The listing builds one solid part. Answer for the finished solid, in the listing's coordinates (mm). A direction names the side the tool comes from. Give positions to 0.01 mm unless a question says otherwise; leave off trailing zeros. Order: outer loops, then holes, each group sorted by start corner. A loop starts at its lowest first (then second) coordinate and runs counter-clockwise, first axis right, second up.
```python
from build123d import *

# Parameters (mm, degrees)
SKETCH2_W                  = 125
SKETCH2_H                  = 95
SKETCH2_R                  = 8
BOSS_EXTRUDE1_DEPTH        = 30
SKETCH3_W                  = 60
SKETCH3_H                  = 60
CUT_EXTRUDE1_DEPTH         = 20
SKETCH4_R                  = 25.5
CUT_EXTRUDE2_DEPTH         = 82.00925873
FILLET1_R                  = 7
FILLET3_R                  = 3
M4_CLEARANCE_HOLE1_D       = 4.5
M6X1_0_TAPPED_HOLE1_REACH  = 119.606
M6X1_0_TAPPED_HOLE1_BORE_R = 2.5
M6X1_0_TAPPED_HOLE2_REACH  = 119.606
M6X1_0_TAPPED_HOLE2_BORE_R = 2.5


with BuildPart() as part:
    # Sketch2 → Boss-Extrude1 (new body)
    with BuildSketch(Plane(origin=(0, 0, 0), x_dir=(1, 0, 0), z_dir=(0, 1, 0))):
        Rectangle(SKETCH2_W, SKETCH2_H)
        with Locations(Location((-44, 29, 0), (0, 0, 270))):
            Circle(SKETCH2_R, mode=Mode.SUBTRACT)
        with Locations(Location((-44, -29, 0), (0, 0, 270))):
            Circle(SKETCH2_R, mode=Mode.SUBTRACT)
        with Locations(Location((44, -29, 0), (0, 0, 270))):
            Circle(SKETCH2_R, mode=Mode.SUBTRACT)
        with Locations(Location((44, 29, 0), (0, 0, 270))):
            Circle(SKETCH2_R, mode=Mode.SUBTRACT)
    extrude(amount=BOSS_EXTRUDE1_DEPTH)

    # Sketch3 → Cut-Extrude1 (cut)
    with BuildSketch(Plane(origin=(0, 30, 0), x_dir=(1, 0, 0), z_dir=(0, 1, 0))):
        Rectangle(SKETCH3_W, SKETCH3_H)
    extrude(amount=-CUT_EXTRUDE1_DEPTH, mode=Mode.SUBTRACT)

    # Sketch4 → Cut-Extrude2 (cut, through all)
    with BuildSketch(Plane(origin=(0, 10, 0), x_dir=(1, 0, 0), z_dir=(0, 1, 0))):
        with Locations(Location((0, 0, 0), (0, 0, 270))):
            Circle(SKETCH4_R)
    extrude(amount=-CUT_EXTRUDE2_DEPTH, mode=Mode.SUBTRACT)

    # Fillet1
    fillet1_edges = [part.edges().sort_by_distance(p)[0] for p in [
        (30, 20, -30),
        (30, 20, 30),
        (-30, 20, 30),
        (-30, 20, -30),
    ]]
    fillet(fillet1_edges, radius=FILLET1_R)

    # Fillet3
    fillet3_edges = [part.edges().sort_by_distance(p)[0] for p in [
        (-62.5, 15, -47.5),
        (62.5, 15, -47.5),
        (62.5, 15, 47.5),
        (-62.5, 15, 47.5),
    ]]
    fillet(fillet3_edges, radius=FILLET3_R)

    # M4 Clearance Hole1 (through all)
    with Locations(Plane(origin=(0, 30, 0), x_dir=(1, 0, 0), z_dir=(0, 1, 0))):
        with Locations((-22, 22), (22, 22), (22, -22), (-22, -22)):
            Hole(M4_CLEARANCE_HOLE1_D / 2)

    # M6x1.0 Tapped Hole1 bore → M6x1.0 Tapped Hole1 (cut, up to next)
    with BuildSketch(Plane.XY.offset(47.5), mode=Mode.PRIVATE) as m6x1_0_tapped_hole1_sk1:
        with Locations((-44, 15)):
            Circle(M6X1_0_TAPPED_HOLE1_BORE_R)
    m6x1_0_tapped_hole1_tool1 = extrude(m6x1_0_tapped_hole1_sk1.sketch, amount=-M6X1_0_TAPPED_HOLE1_REACH, mode=Mode.PRIVATE) & part.part
    # M6x1.0 Tapped Hole1 bore → M6x1.0 Tapped Hole1 (cut, up to next)
    with BuildSketch(Plane.XY.offset(47.5), mode=Mode.PRIVATE) as m6x1_0_tapped_hole1_sk2:
        with Locations((44, 15)):
            Circle(M6X1_0_TAPPED_HOLE1_BORE_R)
    m6x1_0_tapped_hole1_tool2 = extrude(m6x1_0_tapped_hole1_sk2.sketch, amount=-M6X1_0_TAPPED_HOLE1_REACH, mode=Mode.PRIVATE) & part.part
    add(m6x1_0_tapped_hole1_tool1.solids().sort_by_distance((-44, 15, 47.5))[0], mode=Mode.SUBTRACT)
    add(m6x1_0_tapped_hole1_tool2.solids().sort_by_distance((44, 15, 47.5))[0], mode=Mode.SUBTRACT)

    # M6x1.0 Tapped Hole2 bore → M6x1.0 Tapped Hole2 (cut, up to next)
    with BuildSketch(Plane(origin=(0, 0, -47.5), x_dir=(-1, 0, 0), z_dir=(0, 0, -1)), mode=Mode.PRIVATE) as m6x1_0_tapped_hole2_sk1:
        with Locations((-44, 15)):
            Circle(M6X1_0_TAPPED_HOLE2_BORE_R)
    m6x1_0_tapped_hole2_tool1 = extrude(m6x1_0_tapped_hole2_sk1.sketch, amount=-M6X1_0_TAPPED_HOLE2_REACH, mode=Mode.PRIVATE) & part.part
    # M6x1.0 Tapped Hole2 bore → M6x1.0 Tapped Hole2 (cut, up to next)
    with BuildSketch(Plane(origin=(0, 0, -47.5), x_dir=(-1, 0, 0), z_dir=(0, 0, -1)), mode=Mode.PRIVATE) as m6x1_0_tapped_hole2_sk2:
        with Locations((44, 15)):
            Circle(M6X1_0_TAPPED_HOLE2_BORE_R)
    m6x1_0_tapped_hole2_tool2 = extrude(m6x1_0_tapped_hole2_sk2.sketch, amount=-M6X1_0_TAPPED_HOLE2_REACH, mode=Mode.PRIVATE) & part.part
    add(m6x1_0_tapped_hole2_tool1.solids().sort_by_distance((44, 15, -47.5))[0], mode=Mode.SUBTRACT)
    add(m6x1_0_tapped_hole2_tool2.solids().sort_by_distance((-44, 15, -47.5))[0], mode=Mode.SUBTRACT)


solid = part.part
```
1) Straight lines are drawn through the part: probe 1 along X at (y, z) = (15, 42); probe 2 along Z at (x, y) = (-22, 3.5); probe 3 along X at (y, z) = (2, -30). For each, find the intervals that lie inside material, in ascending order.
Geometry says:
probe 1: x = -62.5 to -46.5, -41.5 to 41.5, 46.5 to 62.5
probe 2: z = -47.5 to -24.25, -19.75 to -12.89, 12.89 to 19.75, 24.25 to 47.5
probe 3: x = -62.5 to -51.94, -36.06 to 36.06, 51.94 to 62.5
2) A tool of negligible diameter and unlimited length cuts with its end or side. For faces 4 (the flat face through (30, 20, 0)), 5 (the cylindrical face through (20.962, 4.93, 23.996)), 6 (the cylindrical face through (41.69, 14.04, -42.13)), 7 (the flat face through (-1, 15, 47.5)), 8 (the cylindrical face through (46.31, 14.04, 42.13)), from which of +Z, -Z, +X, -X, +Y, -Y can it reach the whole face along a straight path? Write none if from no direction.
Geometry says:
face 4: +Y
face 5: +Y, -Y
face 6: -Z
face 7: +Z, +X, -X, +Y, -Y
face 8: +Z
3) Find section C-C (z = -32). Write down the section's boundary in (x, y).
Geometry says:
outline: (-62.5, 0) - (-51.42, 0) - (-51.42, 30) - (-62.5, 30) - close; (-36.58, 0) - (36.58, 0) - (36.58, 30) - (-36.58, 30) - close; (51.42, 0) - (62.5, 0) - (62.5, 30) - (51.42, 30) - close
4) Find section A-A (x = 0). Write down the section's boundary in (y, z), then the cut area to 3 significant figures.
Geometry says:
outline: (0, -47.5) - (30, -47.5) - (30, -30) - (10, -30) - (10, -25.5) - (0, -25.5) - close; (0, 25.5) - (10, 25.5) - (10, 30) - (30, 30) - (30, 47.5) - (0, 47.5) - close
area: 1,140 mm2
5) For a pull along Y with two mould halves and no side action, classify faces 1 (the flat face through (-1, 30, 31)), 2 (the cylindrical face through (-41.69, 14.04, 42.13)), 3 (the cylindrical face through (-27.9, 19.9, -28)) as +Y half, -Y half, draft (parallel to the pull), parting line (faces both ways), or undercut.
Geometry says:
face 1: +Y half
face 2: undercut
face 3: draft
6) Find section B-B (y = 19). Write down the section's boundary in (x, z), then the cut area to 3 significant figures.
Geometry says:
outline: (-62.5, -44.5) arc R3 ccw to (-59.5, -47.5) - (59.5, -47.5) arc R3 ccw to (62.5, -44.5) - (62.5, 44.5) arc R3 ccw to (59.5, 47.5) - (-59.5, 47.5) arc R3 ccw to (-62.5, 44.5) - close; hole circle Ø16 at (-44, -29); hole circle Ø16 at (-44, 29); hole (-30, -23) arc R7 ccw to (-23, -30) - (23, -30) arc R7 ccw to (30, -23) - (30, 23) arc R7 ccw to (23, 30) - (-23, 30) arc R7 ccw to (-30, 23) - close; hole circle Ø16 at (44, -29); hole circle Ø16 at (44, 29)
area: 7,510 mm2
7) Find section D-D (x = -44). Write down the section's boundary in (y, z).
Geometry says:
outline: (0, -47.5) - (12.5, -47.5) - (12.5, -37) - (0, -37) - close; (0, -21) - (30, -21) - (30, 21) - (0, 21) - close; (0, 37) - (12.5, 37) - (12.5, 47.5) - (0, 47.5) - close; (17.5, -47.5) - (30, -47.5) - (30, -37) - (17.5, -37) - close; (17.5, 37) - (30, 37) - (30, 47.5) - (17.5, 47.5) - close
8) Given P1, Ø6, axis at x = 4.5, z = 19.5, coming from the -Y side; P2, Ø4.5, axis at x = 44, y = 15, coming from the +Z side, each flat-ended and moving along its own axis, determine where each tip first touches the part or whether it passes through.
Geometry says:
P1: passes through
P2: stops at z = 21.32
